Geometry check sheet. Reference: the model listing, model coordinates, mm. A direction names the side the tool comes from. Coordinates: 2 decimals unless noted, no trailing zeros. Loops run counter-clockwise (first coordinate to the right, second up) from the corner with the lowest first, then second, coordinate; pieces in that order, holes last. Notation, with made-up numbers: M 7.25,80.25 L 50.25,80.25 A25 cw 50.25,116.25 Z; hole C 73,33.5 d11. An arc over 180 degrees is marked long. Use CSV: the item, a comma, the result in double quotes.
Autodesk Fusion 360 part; units mm, degrees
sketch "Sketch1" plane through (0, 0, 0) normal (0, 0, 1) x (1, 0, 0)
  line L0 (0, 0) -> (17, 0)
  line L1 (17, 0) -> (17, -3)
  line L2 (17, -3) -> (17, -5.7)
  line L3 (17, -5.7) -> (17, -12.3)
  line L4 (17, -12.3) -> (15, -12.3)
  line L5 (15, -12.3) -> (15, -0.8)
  line L6 (17, -3) -> (17, -4.35) construction
  line L7 (17, -4.35) -> (16.5, -4.35) construction
  line L8 (17, -3) -> (16.5, -4.35)
  line L9 (16.5, -4.35) -> (17, -5.7)
  line L10 (0, 0) -> (0, -0.8)
  line L11 (0, -0.8) -> (15, -0.8)
  dimension "d1" = 17
  dimension "d2" = 3
  dimension "d4" = 2.7
  dimension "d5" = 6.6
  dimension "d6" = 2
  dimension "d8" = 1.35
  dimension "d9" = 0.5
  dimension "d10" = 15
  dimension "d12" = 17
  dimension "d19" = 0.8
revolve "Revolve1" add sketch "Sketch1" angle 360 about axis through (0, 0, 0) along (0, -1, 0) contours L0 L1 L3 L4 L5 L8 L9 L10 L11
sketch "Sketch2" plane through (0, 0, 0) normal (0, 1, 0) x (-1, 0, 0)
  circle A0 centre (0, 0) radius 17
  circle A1 centre (0, 0) radius 16.575
  circle A2 centre (0, 0) radius 0.75
  dimension "d14" = 34
  dimension "d15" = 33.15
  dimension "d16" = 1.5
extrude "Extrude1" cut sketch "Sketch2" against normal blind 3 contours A2
equation "d15 = d14 - 0.85 mm"
1. Section check B-B, the plane x = 0. Record the cut outline in (y, z).
The answers:
outline,"M -12.3,-17 L -5.7,-17 L -4.35,-16.5 L -3,-17 L 0,-17 L 0,-0.75 L -0.8,-0.75 L -0.8,-15 L -12.3,-15 Z; M -12.3,15 L -0.8,15 L -0.8,0.75 L 0,0.75 L 0,17 L -3,17 L -4.35,16.5 L -5.7,17 L -12.3,17 Z"
2. Thickness scan on line 1 (Z direction, x = 0, y = -8.5); line 2 (Y direction, x = 13.5, z = -3.5); line 3 (X direction, y = -3.75, z = -3). Record the ranges inside material, lowest first. Write a range as [from, to].
The answers:
line 1,"[-17, -15], [15, 17]"
line 2,"[-0.8, 0]"
line 3,"[-16.45, -14.7], [14.7, 16.45]"
3. Release check for a two-part mould opening along Z. For faces 1 (the cylindrical face through (9.139, -1.521, 14.334)), 2 (the flat face through (4, 0, 0)), 3 (the flat face through (0, -0.8, -3)) record: +Z half, -Z half, draft (parallel to the pull), parting line (faces both ways), or undercut.
The answers:
face 1,"parting line"
face 2,"draft"
face 3,"undercut"
4. Set-up check for faces 4 (the cylindrical face through (9.139, -9.046, 14.334)), 5 (the cylindrical face through (-14.985, -6.47, -0.66)): record each of +Z, -Z, +X, -X, +Y, -Y from which the full face is reachable in a straight line by a thin tool's end or side.
The answers:
face 4,"+Y, -Y"
face 5,"-Y"
5. Section check C-C, the plane y = -1.25. Record the cut outline in (x, z), plus the area to 3 significant figures.
The answers:
outline,"C 0,0 d34; hole C 0,0 d30"
area,"201 mm^2"
6. Section check A-A, the plane z = 0. Record the cut outline in (x, y), plus the area to 4 significant figures.
The answers:
outline,"M -17,-12.3 L -15,-12.3 L -15,-0.8 L -0.75,-0.8 L -0.75,0 L -17,0 L -17,-3 L -16.5,-4.35 L -17,-5.7 Z; M 0.75,-0.8 L 15,-0.8 L 15,-12.3 L 17,-12.3 L 17,-5.7 L 16.5,-4.35 L 17,-3 L 17,0 L 0.75,0 Z"
area,"70.65 mm^2"
7. Gauge pin test, flat ends, axial feed: P1, Ø1.5, axis at x = 5.5, z = -11, coming from the -Y side; P2, Ø10, axis at x = -1, z = 13.5, coming from the -Y side; P3, Ø1.5, axis at y = -10.5, z = 10.5, coming from the +X side; P4, Ø1, axis at y = -5, z = -11.5, coming from the +X side. Record the tip position at first contact, or that the pin passes through.
The answers:
P1,"y = -0.8"
P2,"y = -12.3"
P3,"x = 13.93"
P4,"x = 12.68"
